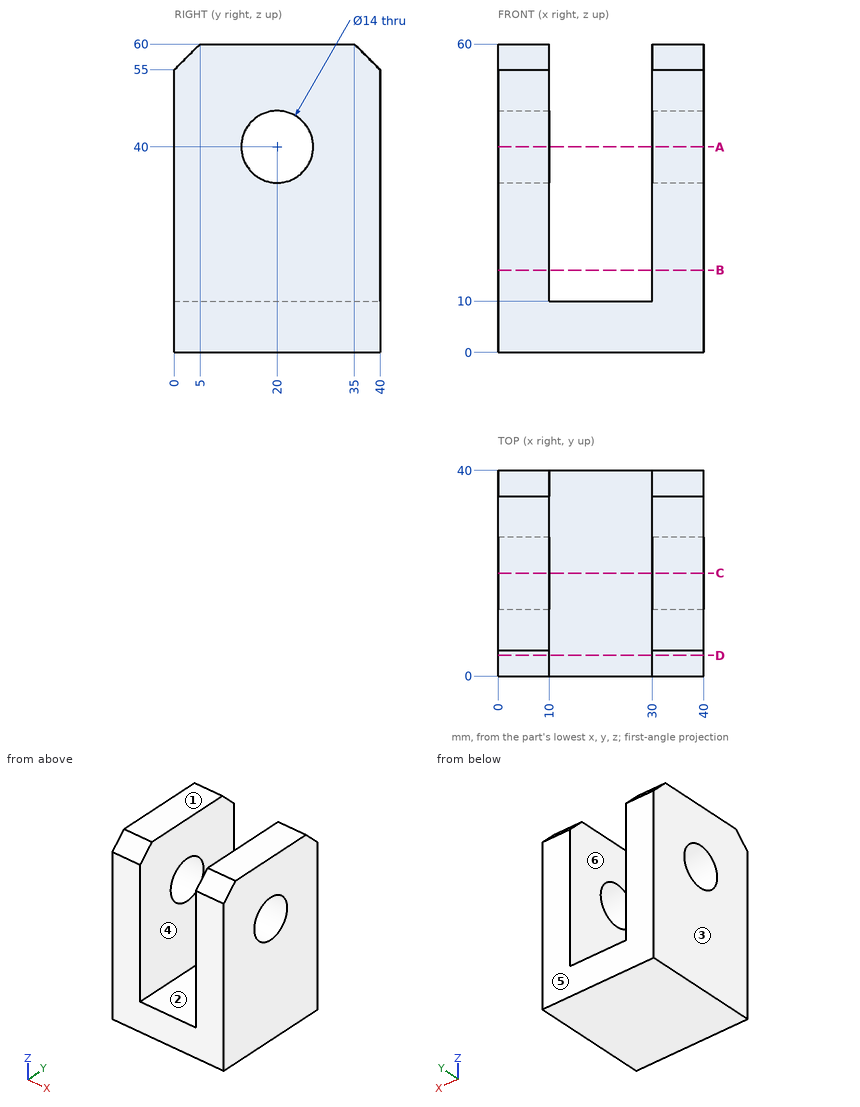
The drawing under review shows one solid part. Ordinate dimensions are in mm from its lowest x, y, z. A direction names the side the tool comes from. Round coordinates to 2 decimals unless told otherwise and drop trailing zeros. Write each loop counter-clockwise with the first axis right and the second up, starting at its lowest first coordinate (ties: lowest second). Pieces come first, ordered by that corner, then holes. Notation, with made-up numbers: (8.25, 43.5) -> (30.25, 43.5) arc R25 ccw to (30.25, 57.5) -> close; hole circle Ø5 at (7, 68.25). An arc over 180 degrees is marked (long way). One line per question, with ' | ' between items. Start each with the question number.
(1) For line 1 along Z through (x, y) = (6, 20); line 2 along X through (y, z) = (23, 21); line 3 along Z through (x, y) = (19, 13.5), list the stretches that pass through material, from the lowest coordinate up. Write a range as from..to.
(2) Insertion check: P1, Ø4, axis at x = 29, y = 15, coming from the +Z side; P2, Ø6, axis at x = 15, y = 6.5, coming from the +Z side. Each pin has a flat end and moves straight along its axis. Give the tip position at first contact, or say it passes through.
(3) Add section A-A, the plane z = 40. Write out the cut boundary in (x, y).
(4) Mouldability with a two-part tool opening along X and no side actions: class the marked faces 3, 4, 5 and 6 as released by +X, released by -X, zero draft, split by the parting line, or undercut.
(5) Add section B-B, the plane z = 16. Write out the cut boundary in (x, y), plus the area to 3 significant figures.
(6) Add section C-C, the plane y = 20. Write out the cut boundary in (x, z), plus the area to 3 significant figures.
(7) Add section D-D, the plane y = 4. Write out the cut boundary in (x, z).
(8) Tool access review of the marked faces 1 and 2: name each direction out of +Z, -Z, +X, -X, +Y, -Y from which nothing blocks a thin tool from reaching the whole face with its end or side.
Answer list:
1) line 1: 0..33, 47..60 | line 2: 0..10, 30..40 | line 3: 0..10
2) P1: z = 60 | P2: z = 10
3) outline: (0, 0) -> (10, 0) -> (10, 13) -> (0, 13) -> close; (0, 27) -> (10, 27) -> (10, 40) -> (0, 40) -> close; (30, 0) -> (40, 0) -> (40, 13) -> (30, 13) -> close; (30, 27) -> (40, 27) -> (40, 40) -> (30, 40) -> close
4) face 3: released by -X | face 4: undercut | face 5: zero draft | face 6: undercut
5) outline: (0, 0) -> (10, 0) -> (10, 40) -> (0, 40) -> close; (30, 0) -> (40, 0) -> (40, 40) -> (30, 40) -> close | area: 800 mm²
6) outline: (0, 0) -> (40, 0) -> (40, 33) -> (30, 33) -> (30, 10) -> (10, 10) -> (10, 33) -> (0, 33) -> close; (0, 47) -> (10, 47) -> (10, 60) -> (0, 60) -> close; (30, 47) -> (40, 47) -> (40, 60) -> (30, 60) -> close | area: 1,120 mm²
7) outline: (0, 0) -> (40, 0) -> (40, 59) -> (30, 59) -> (30, 10) -> (10, 10) -> (10, 59) -> (0, 59) -> close
8) face 1: +Z, +X, -X, +Y, -Y | face 2: +Z, +Y, -Y
